Input: part model. Units: mm. Frame: model coordinates. Face numbers are marked on the shaded views. Round coordinates to 2 decimals unless told otherwise and drop trailing zeros. Loops run counter-clockwise (first coordinate to the right, second up) from the corner with the lowest first, then second, coordinate; pieces in that order, holes last. Notation, with made-up numbers: (87, 29) -> (127, 29) arc R21 ccw to (127, 35) -> close; hole circle Ø8 at (22, 72). An arc over 180 degrees is marked (long way). Answer as a JSON object with one key per item and string values. Group by question number.
Item 1: Draft query along X for the marked faces 1, 2, 3 and 4. Return one class per face: released by +X, released by -X, zero draft, split by the parting line, or undercut.
Item 2: Material intervals for line 1 (Y direction, x = -5, z = -19.35); line 2 (Z direction, x = -5, y = 0.75); line 3 (X direction, y = 2.55, z = -18.25), sorted ascending. Write a range as [from, to].
Item 3: Pin query (flat end, axial travel): pin 1 (0.8 mm diameter, centred on y = 4, z = -2, fed in from +X); pin 2 (0.8 mm diameter, centred on x = -7.5, y = 4, fed in from +Z); pin 3 (1.8 mm diameter, centred on x = -5, z = -5, fed in from +Y). Return the tip coordinate at first contact, or that it passes through.
Item 4: Section query A-A on z = -15.5. Return loops of the section in (x, y), and give its area (3 significant figures).
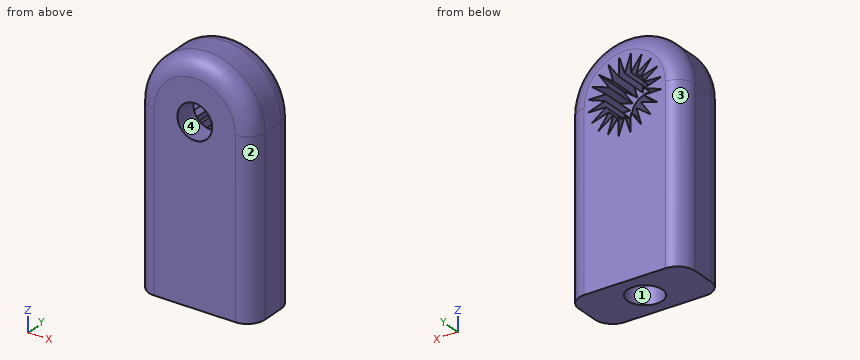
Autodesk Inventor part; units mm, degrees
ref_plane "Work Plane (Clip Axis)" through (0, 2.5, 0) normal (0, 1, 0) x (1, 0, 0)
ref_plane "YZ Plane" through (0, 0, 0) normal (1, 0, 0) x (0, 1, 0)
ref_plane "XZ Plane" through (0, 0, 0) normal (0, 1, 0) x (-1, 0, 0)
sketch "Horn Base Profile" plane through (0, 0, 0) normal (0, 1, 0) x (-1, 0, 0)
  line L0 (0, 0) -> (10, 0) construction
  line L1 (10, 0) -> (10, -20) construction
  line L2 (10, -20) -> (0, -20) construction
  line L3 (0, -20) -> (0, 0) construction
  arc A0 (10, -5) -> (0, -5) centre (5, -5) ccw
  line L4 (10, -5) -> (10, -20)
  line L5 (0, -20) -> (10, -20)
  line L6 (0, -20) -> (0, -5)
  circle A1 centre (5, -5) radius 1.5
  dimension "d0" = 10
  dimension "d1" = 20
  dimension "d2" = 3
extrude "Horn Base" add sketch "Horn Base Profile" along normal blind 2
sketch "Spline Profile" plane through (0, 2, 0) normal (0, 1, 0) x (1, 0, 0)
  line L0 (-10, 20) -> (-10, 5)
  arc A0 (-10, 5) -> (0, 5) centre (-5, 5) ccw
  line L1 (0, 5) -> (0, 20)
  line L2 (0, 20) -> (-10, 20)
  circle A1 centre (-5, 5) radius 1.7 construction
  circle A2 centre (-5, 5) radius 3.2 construction
  line L3 (-5, 5) -> (-5, 3.3) construction
  line L4 (-5, 5) -> (-5.5253, 3.3832) construction
  line L5 (-5, 3.3) -> (-5.5253, 1.8434)
  line L6 (-5.5253, 3.3832) -> (-5.5253, 1.8434)
  line L7 (-4.4747, 3.3832) -> (-4.5242, 1.8356)
  line L8 (-5, 3.3) -> (-4.5242, 1.8356)
  line L9 (-4.0008, 3.6247) -> (-3.5696, 2.1375)
  line L10 (-4.4747, 3.3832) -> (-3.5696, 2.1375)
  line L11 (-3.6247, 4.0008) -> (-2.755, 2.7196)
  line L12 (-4.0008, 3.6247) -> (-2.755, 2.7196)
  line L13 (-3.3832, 4.4747) -> (-2.1602, 3.5249)
  line L14 (-3.6247, 4.0008) -> (-2.1602, 3.5249)
  line L15 (-3.3, 5) -> (-1.8434, 4.4747)
  line L16 (-3.3832, 4.4747) -> (-1.8434, 4.4747)
  line L17 (-3.3832, 5.5253) -> (-1.8356, 5.4758)
  line L18 (-3.3, 5) -> (-1.8356, 5.4758)
  line L19 (-3.6247, 5.9992) -> (-2.1375, 6.4304)
  line L20 (-3.3832, 5.5253) -> (-2.1375, 6.4304)
  line L21 (-4.0008, 6.3753) -> (-2.7196, 7.245)
  line L22 (-3.6247, 5.9992) -> (-2.7196, 7.245)
  line L23 (-4.4747, 6.6168) -> (-3.5249, 7.8398)
  line L24 (-4.0008, 6.3753) -> (-3.5249, 7.8398)
  line L25 (-5, 6.7) -> (-4.4747, 8.1566)
  line L26 (-4.4747, 6.6168) -> (-4.4747, 8.1566)
  line L27 (-5.5253, 6.6168) -> (-5.4758, 8.1644)
  line L28 (-5, 6.7) -> (-5.4758, 8.1644)
  line L29 (-5.9992, 6.3753) -> (-6.4304, 7.8625)
  line L30 (-5.5253, 6.6168) -> (-6.4304, 7.8625)
  line L31 (-6.3753, 5.9992) -> (-7.245, 7.2804)
  line L32 (-5.9992, 6.3753) -> (-7.245, 7.2804)
  line L33 (-6.6168, 5.5253) -> (-7.8398, 6.4751)
  line L34 (-6.3753, 5.9992) -> (-7.8398, 6.4751)
  line L35 (-6.7, 5) -> (-8.1566, 5.5253)
  line L36 (-6.6168, 5.5253) -> (-8.1566, 5.5253)
  line L37 (-6.6168, 4.4747) -> (-8.1644, 4.5242)
  line L38 (-6.7, 5) -> (-8.1644, 4.5242)
  line L39 (-6.3753, 4.0008) -> (-7.8625, 3.5696)
  line L40 (-6.6168, 4.4747) -> (-7.8625, 3.5696)
  line L41 (-5.9992, 3.6247) -> (-7.2804, 2.755)
  line L42 (-6.3753, 4.0008) -> (-7.2804, 2.755)
  line L43 (-5.5253, 3.3832) -> (-6.4751, 2.1602)
  line L44 (-5.9992, 3.6247) -> (-6.4751, 2.1602)
  point P0 (0, 0)
  dimension "d5" = 3.4
  dimension "d6" = 1.5
  dimension "d7" = 18
  dimension "d11" = 360
extrude "Servo Spline Cut" add sketch "Spline Profile" along normal blind 3
ref_plane "Work Plane (Clip Axis)" through (0, 2.5, 0) normal (0, 1, 0) x (1, 0, 0)
sketch "Clip Cut Profile" plane through (0, 2.5, 0) normal (0, 1, 0) x (1, 0, 0)
  line L0 (0, 20) -> (-10, 20) construction
  arc A0 (-10, 5) -> (0, 5) centre (-5, 5) ccw construction
  line L1 (0, 5) -> (0, 20) construction
  line L2 (0, 20) -> (-10, 20) construction
  line L3 (-10, 20) -> (-10, 5) construction
  line L4 (-4.4747, 3.3832) -> (-4.5242, 1.8356) construction
  line L5 (-4.5242, 1.8356) -> (-5, 3.3) construction
  line L6 (-5, 3.3) -> (-5.5253, 1.8434) construction
  line L7 (-5.5253, 1.8434) -> (-5.5253, 3.3832) construction
  line L8 (-5.5253, 3.3832) -> (-6.4751, 2.1602) construction
  line L9 (-6.4751, 2.1602) -> (-5.9992, 3.6247) construction
  line L10 (-5.9992, 3.6247) -> (-7.2804, 2.755) construction
  line L11 (-7.2804, 2.755) -> (-6.3753, 4.0008) construction
  line L12 (-6.3753, 4.0008) -> (-7.8625, 3.5696) construction
  line L13 (-7.8625, 3.5696) -> (-6.6168, 4.4747) construction
  line L14 (-6.6168, 4.4747) -> (-8.1644, 4.5242) construction
  line L15 (-8.1644, 4.5242) -> (-6.7, 5) construction
  line L16 (-6.7, 5) -> (-8.1566, 5.5253) construction
  line L17 (-8.1566, 5.5253) -> (-6.6168, 5.5253) construction
  line L18 (-6.6168, 5.5253) -> (-7.8398, 6.4751) construction
  line L19 (-7.8398, 6.4751) -> (-6.3753, 5.9992) construction
  line L20 (-6.3753, 5.9992) -> (-7.245, 7.2804) construction
  line L21 (-7.245, 7.2804) -> (-5.9992, 6.3753) construction
  line L22 (-5.9992, 6.3753) -> (-6.4304, 7.8625) construction
  line L23 (-6.4304, 7.8625) -> (-5.5253, 6.6168) construction
  line L24 (-5.5253, 6.6168) -> (-5.4758, 8.1644) construction
  line L25 (-5.4758, 8.1644) -> (-5, 6.7) construction
  line L26 (-5, 6.7) -> (-4.4747, 8.1566) construction
  line L27 (-4.4747, 8.1566) -> (-4.4747, 6.6168) construction
  line L28 (-4.4747, 6.6168) -> (-3.5249, 7.8398) construction
  line L29 (-3.5249, 7.8398) -> (-4.0008, 6.3753) construction
  line L30 (-4.0008, 6.3753) -> (-2.7196, 7.245) construction
  line L31 (-2.7196, 7.245) -> (-3.6247, 5.9992) construction
  line L32 (-3.6247, 5.9992) -> (-2.1375, 6.4304) construction
  line L33 (-2.1375, 6.4304) -> (-3.3832, 5.5253) construction
  line L34 (-3.3832, 5.5253) -> (-1.8356, 5.4758) construction
  line L35 (-1.8356, 5.4758) -> (-3.3, 5) construction
  line L36 (-3.3, 5) -> (-1.8434, 4.4747) construction
  line L37 (-1.8434, 4.4747) -> (-3.3832, 4.4747) construction
  line L38 (-3.3832, 4.4747) -> (-2.1602, 3.5249) construction
  line L39 (-2.1602, 3.5249) -> (-3.6247, 4.0008) construction
  line L40 (-3.6247, 4.0008) -> (-2.755, 2.7196) construction
  line L41 (-2.755, 2.7196) -> (-4.0008, 3.6247) construction
  line L42 (-4.0008, 3.6247) -> (-3.5696, 2.1375) construction
  line L43 (-3.5696, 2.1375) -> (-4.4747, 3.3832) construction
  line L44 (0, 5) -> (0, 20) construction
  line L45 (0, 20) -> (-10, 20)
  line L46 (-5, 20) -> (-6.5, 20)
  line L47 (-6.5, 20) -> (-6.5, 18)
  line L48 (-6.5, 18) -> (-5, 18)
  line L49 (-5, 18) -> (-5, 20)
  line L50 (-5, 18) -> (-7, 18)
  line L51 (-7, 18) -> (-7, 16)
  line L52 (-7, 16) -> (-5, 16)
  line L53 (-5, 16) -> (-5, 18)
  point P0 (0, 0)
  point P1 (-6.5, 18)
  dimension "d16" = 1.5
  dimension "d17" = 2
  dimension "d18" = 2
  dimension "d19" = 2
revolve "Fin Clip Cut" cut sketch "Clip Cut Profile" angle 360 about axis through (-5, 2.5, -18) along (0, 0, -1)
fillet "Fillets (Horn Edges)" radius 1.5 6 edges at (-5, 5, 0) (0, 5, -12.5) (-10, 5, -12.5) (-5, 0, 0) (0, 0, -12.5) (-10, 0, -12.5)
properties part number "flipper_robot_v2_servo_adapter"
Solved:
{
 "1": {"face 1": "undercut", "face 2": "released by +X", "face 3": "released by -X", "face 4": "undercut"},
 "2": {"line 1": "[0, 1], [4, 5]", "line 2": "[-20, -18], [-16, -6.5], [-3.5, -0.2]", "line 3": "[-10, -6.5], [-3.5, 0]"},
 "3": {"pin 1": "x = -0.8", "pin 2": "z = -0.52", "pin 3": "through"},
 "4": {"outline": "(-10, 1.5) arc R1.5 ccw to (-8.5, 0) -> (-1.5, 0) arc R1.5 ccw to (0, 1.5) -> (0, 3.5) arc R1.5 ccw to (-1.5, 5) -> (-8.5, 5) arc R1.5 ccw to (-10, 3.5) -> close", "area": "48.1 mm²"}
}
